from build123d import *

# Parameters (mm, degrees)
BOSS_EXTRUDE1_DEPTH = 10
SKETCH2_R           = 1.5
CUT_EXTRUDE1_DEPTH  = 10


with BuildPart() as part:
    # Sketch1 → Boss-Extrude1 (new body)
    with BuildSketch(Plane(origin=(0, 0, 0), x_dir=(1, 0, 0), z_dir=(0, 1, 0))):
        Polygon((18, -9), (18, -18), (-18, -18), (-18, 18), (18, 18), (18, 9), (34, 9), (34, -9), align=None)
    extrude(amount=BOSS_EXTRUDE1_DEPTH)

    # Sketch2 → Cut-Extrude1 (cut)
    with BuildSketch(Plane(origin=(0, 10, 0), x_dir=(1, 0, 0), z_dir=(0, 1, 0))):
        with Locations(Location((-15.25, 15.25, 0), (0, 0, 270))):
            Circle(SKETCH2_R)
        with Locations(Location((15.25, 15.25, 0), (0, 0, 270))):
            Circle(SKETCH2_R)
        with Locations(Location((-15.25, -15.25, 0), (0, 0, 270))):
            Circle(SKETCH2_R)
        with Locations(Location((15.25, -15.25, 0), (0, 0, 270))):
            Circle(SKETCH2_R)
    extrude(amount=-CUT_EXTRUDE1_DEPTH, mode=Mode.SUBTRACT)


solid = part.part
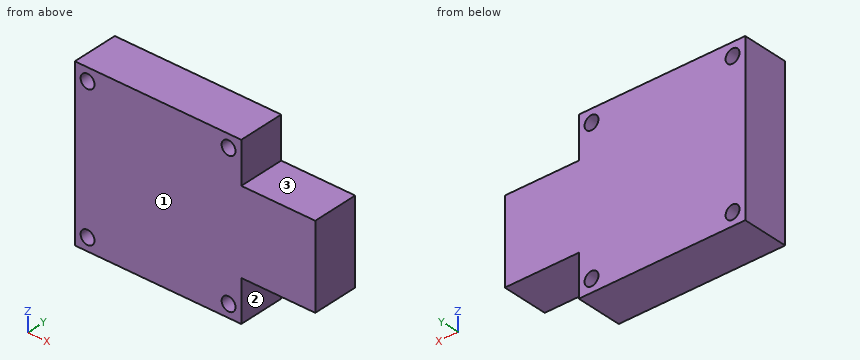
Could you check a few things on this model? Use its own coordinates, in mm. Face numbers are marked on the shaded views. A direction names the side the tool comes from. Round coordinates to 2 decimals unless told otherwise and drop trailing zeros. Write each loop counter-clockwise with the first axis right and the second up, starting at its lowest first coordinate (ties: lowest second). Pieces come first, ordered by that corner, then holes. Notation, with made-up numbers: (-6.75, 5.5) -> (19.25, 5.5) arc R27 cw to (19.25, 36.5) -> close; hole circle Ø1 at (7.25, -9). An arc over 180 degrees is marked (long way). Use a Markdown table: item, result.
1. If we section it at D-D (x = 28): List the corners of the cut face in (y, z) for me, then the cut area to 3 significant figures.
Answer key:
| item | result |
|---|---|
| outline | (0, -9) -> (10, -9) -> (10, 9) -> (0, 9) -> close |
| area | 180 mm^2 |
2. For pin 1 Ø2.5 at (y, z) = (5.5, -11.5) entering from +X; pin 2 Ø5 at (x, y) = (24, 4) entering from -Z, each with a flat end and sliding along its axis, tell me the tip position at first contact or that it passes through.
Answer key:
| item | result |
|---|---|
| pin 1 | stops at x = 18 |
| pin 2 | stops at z = -9 |
3. If we section it at C-C (y = 3.5): List the corners of the cut face in (x, z) for me, then the cut area to 3 significant figures.
Answer key:
| item | result |
|---|---|
| outline | (-18, -18) -> (18, -18) -> (18, -9) -> (34, -9) -> (34, 9) -> (18, 9) -> (18, 18) -> (-18, 18) -> close; hole circle Ø3 at (-15.25, -15.25); hole circle Ø3 at (-15.25, 15.25); hole circle Ø3 at (15.25, -15.25); hole circle Ø3 at (15.25, 15.25) |
| area | 1,560 mm^2 |
4. If we section it at A-A (z = 15.25): List the corners of the cut face in (x, y) for me.
Answer key:
| item | result |
|---|---|
| outline | (-18, 0) -> (-16.75, 0) -> (-16.75, 10) -> (-18, 10) -> close; (-13.75, 0) -> (13.75, 0) -> (13.75, 10) -> (-13.75, 10) -> close; (16.75, 0) -> (18, 0) -> (18, 10) -> (16.75, 10) -> close |
5. If we section it at B-B (x = -15.25): List the corners of the cut face in (y, z) for me, then the cut area to 3 significant figures.
Answer key:
| item | result |
|---|---|
| outline | (0, -18) -> (10, -18) -> (10, -16.75) -> (0, -16.75) -> close; (0, -13.75) -> (10, -13.75) -> (10, 13.75) -> (0, 13.75) -> close; (0, 16.75) -> (10, 16.75) -> (10, 18) -> (0, 18) -> close |
| area | 300 mm^2 |
6. Please list where these lines run through material, in increasing order: probe 1 along X at (y, z) = (6.5, -15.25); probe 2 along X at (y, z) = (6.5, 9.5); probe 3 along Z at (x, y) = (20, 9.75).
Answer key:
| item | result |
|---|---|
| probe 1 | x = -18 to -16.75, -13.75 to 13.75, 16.75 to 18 |
| probe 2 | x = -18 to 18 |
| probe 3 | z = -9 to 9 |
7. Which directions (+Z, -Z, +X, -X, +Y, -Y) give clear straight access to the entire face, cutting with the end or side of a thin tool? Please do the marked faces 1, 2 and 3.
Answer key:
| item | result |
|---|---|
| face 1 | +Z, -Z, +X, -X, -Y |
| face 2 | -Z, +X, +Y, -Y |
| face 3 | +Z, +X, +Y, -Y |
